from build123d import *

# Parameters (mm, degrees)
F0_R     = 42.5
F1_DEPTH = 19
F2_W     = 7
F2_H     = 4
F4_R     = 30
F5_DEPTH = 16
F6_R     = 27
F7_DEPTH = 12


# Not quite as in the source:
# - a fillet or chamfer that OpenCascade refuses, or shapes differently, is made with other operations: its cross-section is extruded or revolved along the edge and cut away or added


with BuildPart() as f1:
    # F0 (on Front) → F1 (new body)
    with BuildSketch(Plane.XZ):
        Circle(F0_R)
    extrude(amount=F1_DEPTH)

    # F2 (on Right) → F3 (revolve, cut)
    with BuildSketch(Plane.YZ):
        with Locations((-7.9, 40.5)):
            Rectangle(F2_W, F2_H)
    revolve(axis=Axis((0, 0, 0), (0, 1, 0)), mode=Mode.SUBTRACT)

    # F4 (on face) → F5 (join)
    with BuildSketch(Plane(origin=(0, 0, 0), x_dir=(-1, 0, 0), z_dir=(0, 1, 0))):
        Circle(F4_R)
    extrude(amount=F5_DEPTH)

    # F6 (on face) → F7 (join)
    with BuildSketch(Plane(origin=(0, 16, 0), x_dir=(-1, 0, 0), z_dir=(0, 1, 0))):
        Circle(F6_R)
    extrude(amount=F7_DEPTH)

    # F8 (on Top) → F9 (revolve, cut)
    with BuildSketch(Plane.XY):
        Polygon((-30, 16), (-30, 0), (-28.6875, 7), (-18.6875, 7), (-18.6875, 16), align=None)
    revolve(axis=Axis((0, 23.2052635401, 0), (0, 1, 0)), mode=Mode.SUBTRACT)

    # F10: chamfer of 1 on 8 edges, made by hand

    # F10_s1 → F10_t2 (revolve, cut)
    with BuildSketch(Plane.XY):
        Polygon((42.5, -3.4), (41.5, -4.4), (42.5, -4.4), align=None)
    revolve(axis=Axis((0, -4.4, 0), (0, 1, 0)), mode=Mode.SUBTRACT)

    # F10_s3 → F10_t4 (revolve, cut)
    with BuildSketch(Plane.XY):
        Polygon((41.5, -11.4), (42.5, -12.4), (42.5, -11.4), align=None)
    revolve(axis=Axis((0, -11.4, 0), (0, 1, 0)), mode=Mode.SUBTRACT)

    # F10_s5 → F10_t6 (revolve, cut)
    with BuildSketch(Plane.XY):
        Polygon((42.5, -18), (41.5, -19), (42.5, -19), align=None)
    revolve(axis=Axis((0, -19, 0), (0, -1, 0)), mode=Mode.SUBTRACT)

    # F10_s7 → F10_t8 (revolve, cut)
    with BuildSketch(Plane.XY):
        Polygon((42.5, -1), (41.5, 0), (42.5, 0), align=None)
    revolve(axis=Axis((0, 0, 0), (0, -1, 0)), mode=Mode.SUBTRACT)

    # F10_s9 → F10_t10 (revolve, cut)
    with BuildSketch(Plane.XY):
        Polygon((-28.8404458997, 6.1842885351), (-27.8575737127, 7), (-28.6875, 7), align=None)
    revolve(axis=Axis((0, 7, 0), (0, 1, 0)), mode=Mode.SUBTRACT)

    # F10_s11 → F10_t12 (revolve, cut)
    with BuildSketch(Plane.XY):
        Polygon((-26, 16), (-27, 17), (-27, 16), align=None)
    revolve(axis=Axis((0, 16, 0), (0, 1, 0)), mode=Mode.SUBTRACT)

    # F10_s13 → F10_t14 (revolve, cut)
    with BuildSketch(Plane.XY):
        Polygon((-27, 27), (-26, 28), (-27, 28), align=None)
    revolve(axis=Axis((0, 28, 0), (0, 1, 0)), mode=Mode.SUBTRACT)


solid = f1.part
Read the model definition and answer for the solid it produces. Units are mm, in the model's axes. A direction names the side the tool comes from. Coordinates: 2 decimals unless noted, no trailing zeros. Write each loop counter-clockwise with the first axis right and the second up, starting at its lowest first coordinate (ties: lowest second). Pieces come first, ordered by that corner, then holes. Notation, with made-up numbers: M 0.5,-37 L 37.5,-37 A28 cw 37.5,-5 Z; hole C 1.5,14.5 d11. An arc over 180 degrees is marked long. Use a Markdown table: item, result.
Q1. Straight lines are drawn through the part: L1, parallel to Y at x = -21, z = 7; L2, parallel to Y at x = -30.5, z = 7; L3, parallel to Z at x = -9, y = 15.5. For each, find the intervals that lie inside material, in ascending order. Write a range as [from, to].
Answer block:
| item | result |
|---|---|
| L1 | y = [-19, 7], [16, 28] |
| L2 | y = [-19, 0] |
| L3 | z = [-16.38, 16.38] |
Q2. The part is cut by section A-A, the plane y = 9. Write down the section's boundary in (x, z) (1 decimal), then the cut area to 3 significant figures.
Answer block:
| item | result |
|---|---|
| outline | C 0,0 d37.4 |
| area | 1,100 mm2 |
Q3. Each of these flat-tipped pins is pushed along its axis until it touches: pin 1 Ø8 at (x, y) = (30, 13.5) entering from -Z; pin 2 Ø5 at (x, y) = (-3.5, -1) entering from +Z; pin 3 Ø1 at (y, z) = (-14, 2.5) entering from -X; pin 4 Ø1 at (x, y) = (13.5, -10) entering from +Z. Where does it stop, or does it pass through?
Answer block:
| item | result |
|---|---|
| pin 1 | passes through |
| pin 2 | stops at z = 42.49 |
| pin 3 | stops at x = -42.45 |
| pin 4 | stops at z = 36.24 |
Q4. Determine the mould class of faces 1 (the face through (-1, -19, 1)), 2 (the face through (0, 28, 0)), 3 (the face through (5.85, 21.93, -26.36)), 4 (the face through (-18, 7, -6)) for opening direction Y: released by +Y, released by -Y, zero draft, split by the parting line, or undercut.
Answer block:
| item | result |
|---|---|
| face 1 | released by -Y |
| face 2 | released by +Y |
| face 3 | zero draft |
| face 4 | undercut |
Q5. Which of the six approach directions +Z, -Z, +X, -X, +Y, -Y give full straight-line access (tool end or side, diameter ignored) to faces 5 (the face through (-18, 16, 6)), 6 (the face through (-33.727, -15.161, -25.861)), 7 (the face through (27.5, 0, 12.5))?
Answer block:
| item | result |
|---|---|
| face 5 | none |
| face 6 | +Y, -Y |
| face 7 | +Y |
Q6. The part is cut by section B-B, the plane y = -10. Write down the section's boundary in (x, z).
Answer block:
| item | result |
|---|---|
| outline | C 0,0 d77 |
